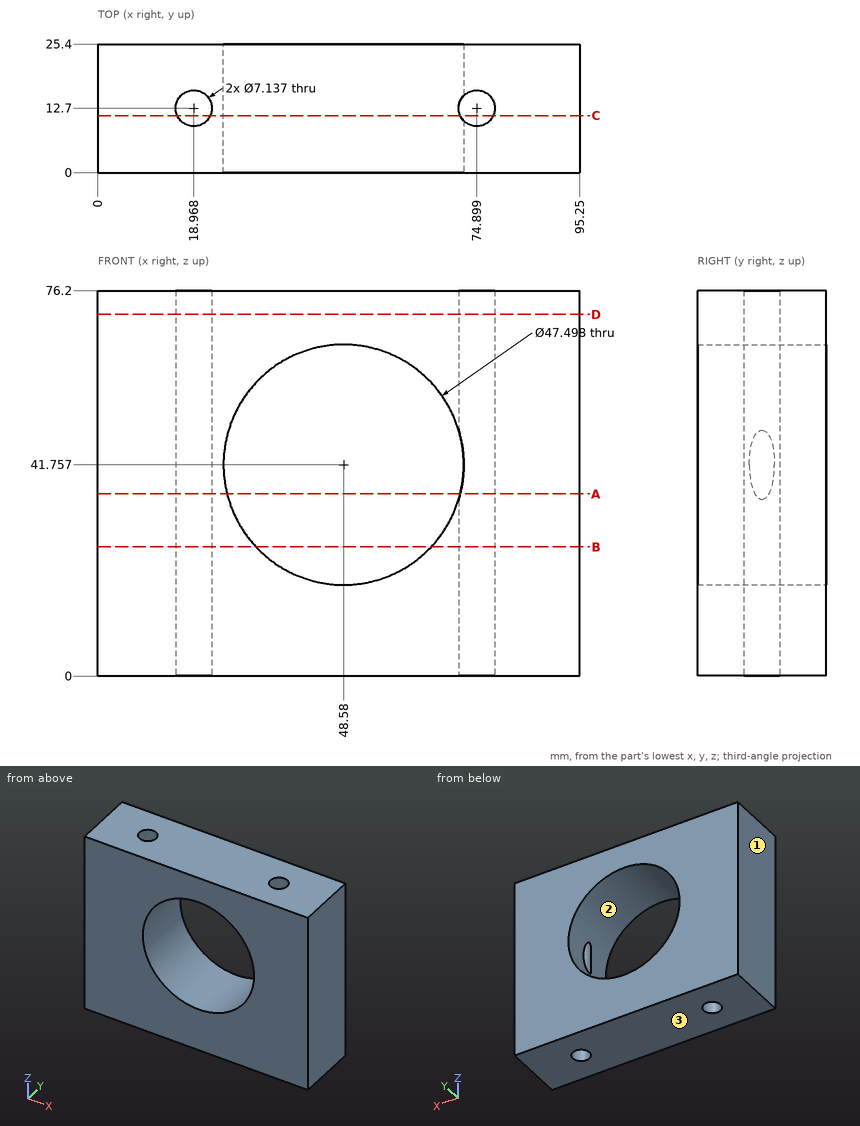
Here's the drawing with two shaded views (mm, measured from the low corner). I have some questions. Coordinates: 2 decimals unless noted, no trailing zeros. Loops run counter-clockwise (first coordinate to the right, second up) from the corner with the lowest first, then second, coordinate; pieces in that order, holes last. Notation, with made-up numbers: (-25, 68.25) -> (26, 68.25) arc R31 cw to (26, 99.25) -> close; hole circle Ø5 at (-9.75, 62.25). An arc over 180 degrees is marked (long way). Answer as a JSON object with one key per item and string values.
1) Thinking about a two-plate mould opening in X: for the marked faces 1, 2 and 3, which applies, pulls with the +X half, pulls with the -X half, needs draft (parallel to the pull), parting line crosses it, or undercut?
Results:
{"face 1": "pulls with the -X half", "face 2": "undercut", "face 3": "needs draft"}
2) Imagine slicing it at D-D (z = 71.5). Please give me the cut outline in (x, y).
Results:
{"outline": "(0, 0) -> (95.25, 0) -> (95.25, 25.4) -> (0, 25.4) -> close; hole circle Ø7.14 at (18.97, 12.7); hole circle Ø7.14 at (74.9, 12.7)"}
3) Imagine slicing it at A-A (z = 36). Please give me the cut outline in (x, y), then the cut area to 3 significant figures.
Results:
{"outline": "(0, 0) -> (25.54, 0) -> (25.54, 25.4) -> (0, 25.4) -> close; (71.62, 0) -> (95.25, 0) -> (95.25, 25.4) -> (71.62, 25.4) -> (71.62, 14.11) arc R3.57 cw (long way) to (71.62, 11.29) -> close; hole circle Ø7.14 at (18.97, 12.7)", "area": "1,170 mm^2"}
4) For P1, Ø8, axis at y = 21, z = 52.5, coming from the -X side, with a flat end and sliding along its axis, tell me the tip position at first contact or that it passes through.
Results:
{"P1": "stops at x = 0"}
5) Imagine slicing it at C-C (y = 11.25). Count the separate pieces of the cut face and the enclosed holes in it, then the cut area to 3 significant figures.
Results:
{"separate pieces": "3", "enclosed holes": "0", "area": "4,500 mm^2"}
6) If I drill on line 1 (Y direction, x = 77.5, z = 71) (1 decimal); line 2 (Y direction, x = 75.5, z = 12); line 3 (X direction, y = 19, z = 48.5), over which ranges is the centre line in solid material (lowest first)?
Results:
{"line 1": "y = 0 to 10.3, 15.1 to 25.4", "line 2": "y = 0 to 9.18, 16.22 to 25.4", "line 3": "x = 0 to 25.81, 71.35 to 95.25"}
7) Imagine slicing it at B-B (z = 25.5). Please give me the cut outline in (x, y).
Results:
{"outline": "(0, 0) -> (31.27, 0) -> (31.27, 25.4) -> (0, 25.4) -> close; (65.89, 0) -> (95.25, 0) -> (95.25, 25.4) -> (65.89, 25.4) -> close; hole circle Ø7.14 at (18.97, 12.7); hole circle Ø7.14 at (74.9, 12.7)"}
